```python
from build123d import *

# Parameters (mm, degrees)
SKETCH_1_R      = 5
SKETCH_1_R_2    = 2.5
EXTRUDE_1_DEPTH = 6


with BuildPart() as part:
    # 스케치1 → 보스-돌출1 (new body)
    # profile 1 of 2: a face of its own
    with BuildSketch(Plane.XY):
        Circle(SKETCH_1_R)
        Circle(SKETCH_1_R_2, mode=Mode.SUBTRACT)
    # profile 2 of 2: a face of its own
    with BuildSketch(Plane.XY):
        with BuildLine():
            Line((15.232380882, 5), (0, 5))
            ThreePointArc((0, 5), (3.535533906, 3.535533906), (5, 0))
            ThreePointArc((5, 0), (0, -5), (-5, 0))
            Line((-5, 0), (-5, -10.728628998))
            Line((-5, -10.728628998), (0.389281966, -16.117910964))
            Line((0.389281966, -16.117910964), (0.389281966, -32.993510276))
            Line((0.389281966, -32.993510276), (1.140402407, -34.2331528))
            Line((1.140402407, -34.2331528), (1.140402407, -37.017391391))
            Line((1.140402407, -37.017391391), (3.188469753, -35.776432632))
            Line((3.188469753, -35.776432632), (10.435477501, -6.24434983))
            Line((10.435477501, -6.24434983), (20.74109717, 0))
            Line((20.74109717, 0), (20.74109717, 5.58326458))
            Line((20.74109717, 5.58326458), (18.231984896, 8.092376853))
            Line((18.231984896, 8.092376853), (15.340369062, 8.092376853))
            Line((15.340369062, 8.092376853), (15.232380882, 5))
        make_face()
    extrude(amount=EXTRUDE_1_DEPTH)


solid = part.part
```
For this review, take the finished solid that the model builds, in its own axes (mm). A direction names the side the tool comes from. Round coordinates to 2 decimals unless told otherwise and drop trailing zeros. Order: outer loops, then holes, each group sorted by start corner. A loop starts at its lowest first (then second) coordinate and runs counter-clockwise, first axis right, second up. Notation, with made-up numbers: (75.5, 17) -> (128.5, 17) arc R7 ccw to (128.5, 26) -> close; hole circle Ø6 at (67.5, 14.25). An arc over 180 degrees is marked (long way). Use a Markdown table: item, result.
Item 1: For pin 1 (1.5 mm diameter, centred on x = 1, z = 3, fed in from -Y); pin 2 (1.5 mm diameter, centred on y = -5.5, z = 2, fed in from +X); pin 3 (3 mm diameter, centred on x = 12.5, z = 4.5, fed in from -Y), all flat-tipped, find the tip position at first contact; note any pin that passes through.
Resolved:
| item | result |
|---|---|
| pin 1 | stops at y = -37.02 |
| pin 2 | stops at x = 12.9 |
| pin 3 | stops at y = -5.9 |
Item 2: Take a section at A-A (z = 4.7). State the section outline as (x, y) points.
Resolved:
| item | result |
|---|---|
| outline | (-5, -10.73) -> (0.39, -16.12) -> (0.39, -32.99) -> (1.14, -34.23) -> (1.14, -37.02) -> (3.19, -35.78) -> (10.44, -6.24) -> (20.74, 0) -> (20.74, 5.58) -> (18.23, 8.09) -> (15.34, 8.09) -> (15.23, 5) -> (0, 5) arc R5 ccw to (-5, 0) -> close; hole circle Ø5 at (0, 0) |
Item 3: Take a section at C-C (x = 13). State the section outline as (y, z) points, plus the area to 3 significant figures.
Resolved:
| item | result |
|---|---|
| outline | (-4.69, 0) -> (5, 0) -> (5, 6) -> (-4.69, 6) -> close |
| area | 58.1 mm² |
Item 4: Draft analysis for pull direction X (two halves, no side actions). For faces 1 (the flat face through (5, -9, 6)), 2 (the cylindrical face through (-0.54, -2.44, 2.96)), 3 (the flat face through (6.76, -21.22, 2.96)), state which applies: +X half, -X half, draft (parallel to the pull), parting line (faces both ways), or undercut.
Resolved:
| item | result |
|---|---|
| face 1 | draft |
| face 2 | undercut |
| face 3 | +X half |
Item 5: Machinability: for faces 4 (the flat face through (8, 5, 3)), 5 (the flat face through (2.15, -36.406, 2.958)), 6 (the flat face through (1.14, -36, 3)), which of the approach directions +Z, -Z, +X, -X, +Y, -Y give a long, thin tool a straight path to every point of the face, cutting with its end or side? Answer none if there is none.
Resolved:
| item | result |
|---|---|
| face 4 | +Z, -Z, -X, +Y |
| face 5 | +Z, -Z, +X, -Y |
| face 6 | +Z, -Z, -X, -Y |
Item 6: For line 1 along Y through (x, z) = (-1, 2.5); line 2 along Y through (x, z) = (0, 4.35); line 3 along Y through (x, z) = (18.25, 1.45), list the stretches that pass through material, from the lowest coordinate up. Write a range as [from, to].
Resolved:
| item | result |
|---|---|
| line 1 | y = [-14.73, -2.29], [2.29, 4.9] |
| line 2 | y = [-15.73, -2.5], [2.5, 5] |
| line 3 | y = [-1.51, 8.07] |
Item 7: Take a section at B-B (y = -30.5). State the section outline as (x, z) points, plus the area to 3 significant figures.
Resolved:
| item | result |
|---|---|
| outline | (0.39, 0) -> (4.48, 0) -> (4.48, 6) -> (0.39, 6) -> close |
| area | 24.6 mm² |
